Geometry check sheet. Reference: drawing and pictorial views, mm from the part's lowest x, y, z. A direction names the side the tool comes from. Coordinates: 2 decimals unless noted, no trailing zeros. Loops run counter-clockwise (first coordinate to the right, second up) from the corner with the lowest first, then second, coordinate; pieces in that order, holes last. Notation, with made-up numbers: (-7.75, 3) -> (49.25, 3) arc R16 cw to (49.25, 32) -> close; hole circle Ø3 at (-37.5, 4.25). An arc over 180 degrees is marked (long way). Answer as a JSON object with one key per item and string values. Group by question number.
Q1. Scan lines: L1, parallel to Z at x = 41.5, y = 64; L2, parallel to X at y = 42.5, z = 81.5 (1 decimal); L3, parallel to Y at x = 98, z = 45. Record each from-to range of solid material in increasing order.
Q2. Cross-section at B-B on y = 56. Record the boundary of the cut face in (x, z) (1 decimal).
Q3. Gauge pin test, flat ends, axial feed: pin 1 Ø10 at (y, z) = (33, 70.5) entering from +X; pin 2 Ø20.5 at (x, y) = (124.5, 15.5) entering from +Z; pin 3 Ø10 at (x, y) = (127, 10.5) entering from -Z; pin 4 Ø12 at (x, z) = (43.5, 70.5) entering from -Y. Record the tip position at first contact, or that the pin passes through.
Q4. Cross-section at C-C on x = 46.5. Record the boundary of the cut face in (y, z), and give its area (3 significant figures).
Q5. Set-up check for the marked faces 1, 2 and 3: record each of +Z, -Z, +X, -X, +Y, -Y from which the full face is reachable in a straight line by a thin tool's end or side.
Q6. Cross-section at A-A on z = 43.5. Record the boundary of the cut face in (x, y) (1 decimal).
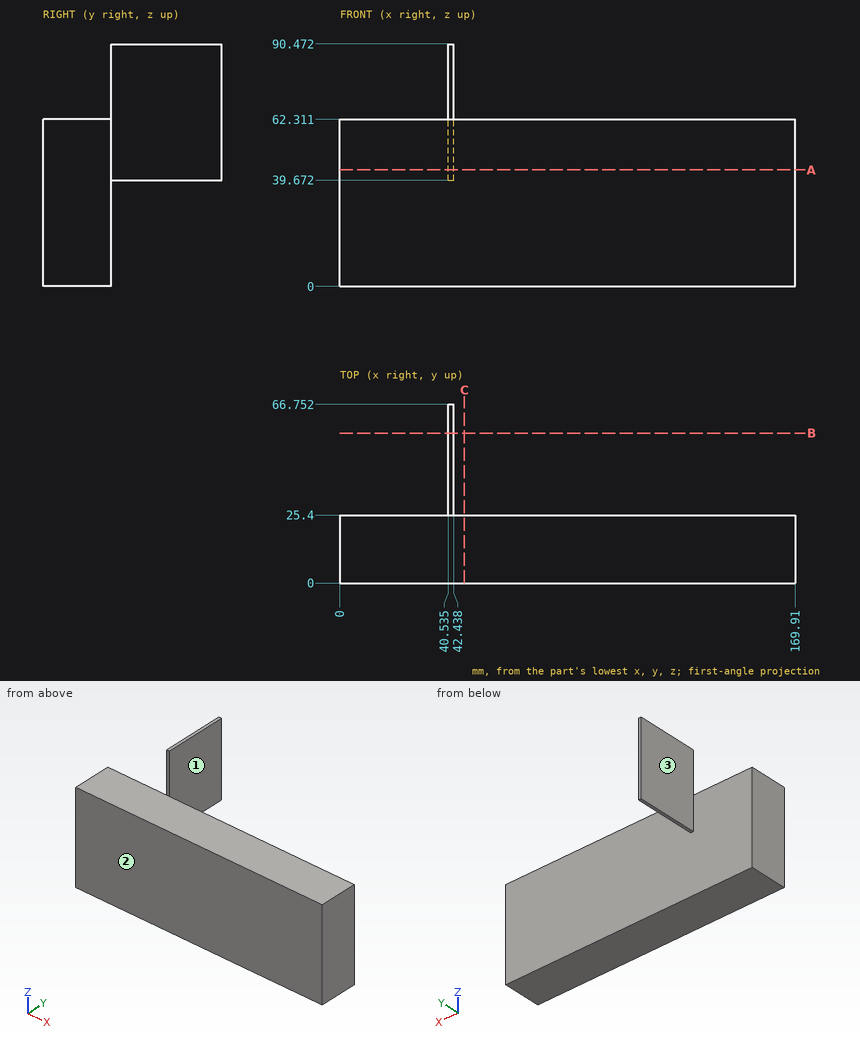
Computed values:
{
 "1": {"L1": "z = 39.67 to 90.47", "L2": "x = 40.5 to 42.4", "L3": "y = 0 to 25.4"},
 "2": {"outline": "(40.5, 39.7) -> (42.4, 39.7) -> (42.4, 90.5) -> (40.5, 90.5) -> close"},
 "3": {"pin 1": "stops at x = 42.44", "pin 2": "stops at z = 62.31", "pin 3": "stops at z = 0", "pin 4": "stops at y = 25.4"},
 "4": {"outline": "(0, 0) -> (25.4, 0) -> (25.4, 62.31) -> (0, 62.31) -> close", "area": "1,580 mm²"},
 "5": {"face 1": "+Z, -Z, +X, +Y", "face 2": "+Z, -Z, +X, -X, -Y", "face 3": "+Z, -Z, -X, +Y"},
 "6": {"outline": "(0, 0) -> (169.9, 0) -> (169.9, 25.4) -> (42.4, 25.4) -> (42.4, 66.8) -> (40.5, 66.8) -> (40.5, 25.4) -> (0, 25.4) -> close"}
}
